from build123d import *

# Parameters (mm, degrees)
BOSS_EXTRUDE1_DEPTH = 3.81


with BuildPart() as part:
    # Sketch1 → Boss-Extrude1 (new body)
    with BuildSketch(Plane.XY):
        with BuildLine():
            Line((66.385047378, -20.797940286), (39.917099653, -20.797940286))
            Line((39.917099653, -20.797940286), (-33.436952622, -20.797940286))
            Line((-33.436952622, -20.797940286), (-33.436952622, -68.922192769))
            Line((-33.436952622, -68.922192769), (-33.436952622, -77.344690286))
            Line((-33.436952622, -77.344690286), (-20.736952622, -77.344690286))
            Line((-20.736952622, -77.344690286), (-20.736952622, -82.107190286))
            Line((-20.736952622, -82.107190286), (-33.436952622, -82.107190286))
            Line((-33.436952622, -82.107190286), (-33.436952622, -140.177940286))
            Line((-33.436952622, -140.177940286), (2.135249773, -140.177940286))
            Line((2.135249773, -140.177940286), (66.385047378, -140.177940286))
            ThreePointArc((66.385047378, -140.177940286), (68.181098603, -139.43399151), (68.925047378, -137.637940286))
            Line((68.925047378, -137.637940286), (68.925047378, -80.487940286))
            Line((68.925047378, -80.487940286), (68.925047378, -23.337940286))
            ThreePointArc((68.925047378, -23.337940286), (68.181098603, -21.541889062), (66.385047378, -20.797940286))
        make_face()
    extrude(amount=BOSS_EXTRUDE1_DEPTH)


solid = part.part
The listing builds one solid part. Answer for the finished solid, in the listing's coordinates (mm). A direction names the side the tool comes from. Coordinates: 2 decimals unless noted, no trailing zeros. Loops run counter-clockwise (first coordinate to the right, second up) from the corner with the lowest first, then second, coordinate; pieces in that order, holes last. Notation, with made-up numbers: (11.5, 8) -> (29.5, 8) arc R20 cw to (29.5, 41) -> close; hole circle Ø10 at (50, -13). An arc over 180 degrees is marked (long way). Write item = value, one per line. Start each with the question number.
1) The mould has two halves that part along Y. Classify faces 3 (the face through (-27, -82.107, 2)), 4 (the face through (68.925, -81, 2)), 5 (the face through (16, -140.178, 2)), 6 (the face through (-20.737, -80, 2)): released by +Y, released by -Y, zero draft, split by the parting line, or undercut.
2) A tool of negligible diameter and unlimited length cuts with its end or side. For faces 1 (the face through (17, -20.798, 2)), 2 (the face through (-27, -77.345, 2)), from which of +Z, -Z, +X, -X, +Y, -Y can it reach the whole face along a straight path? Write none if from no direction.
3) A cutting plane is placed at A-A (x = -24). Give the vertices of the cut face in (y, z).
4) Given pin 1 Ø4 at (x, y) = (-19.5, -111.5) entering from -Z; pin 2 Ø1.9 at (y, z) = (-80.5, 1) entering from -X, each flat-ended and moving along its own axis, determine where each tip first touches the part or whether it passes through.
Responses:
q1.face_3 = undercut
q1.face_4 = zero draft
q1.face_5 = released by -Y
q1.face_6 = undercut
q2.face_1 = +Z, -Z, +X, -X, +Y
q2.face_2 = +Z, -Z, -X
q3.outline = (-140.18, 0) -> (-82.11, 0) -> (-82.11, 3.81) -> (-140.18, 3.81) -> close; (-77.34, 0) -> (-20.8, 0) -> (-20.8, 3.81) -> (-77.34, 3.81) -> close
q4.pin_1 = 0
q4.pin_2 = -20.74
